Part model, mm, in its own coordinate system. A direction names the side the tool comes from. Give positions to 0.01 mm unless a question says otherwise; leave off trailing zeros. Write each loop counter-clockwise with the first axis right and the second up, starting at its lowest first coordinate (ties: lowest second). Pieces come first, ordered by that corner, then holes. Notation, with made-up numbers: M -33.5,36 L -11.5,36 A12 ccw -11.5,49 Z; hole C 13,-10.5 d1. An arc over 180 degrees is marked long. Use CSV: the item, a comma, the result in double quotes. Start each with the question number.
1. Band-saw the part on A-A, the plane z = -47.5. List the corners of the cut face in (x, y), then the cut area to 3 significant figures.
2. Mould opens along Z. For faces 1 (the face through (-76.986, 2.465, 77.297)), 2 (the face through (-1, 2, 95)), 3 (the face through (-88.866, 2.535, 73.953)), 4 (the face through (-1, 2, -95)) say: pulls with the +Z half, pulls with the -Z half, needs draft (parallel to the pull), parting line crosses it, or undercut.
3. Band-saw the part on B-B, the plane x = -54.5. List the corners of the cut face in (y, z).
4. Band-saw the part on C-C, the plane y = 4.05. Count the separate pieces of the cut face and the enclosed holes in it, then the cut area to 3 significant figures.
5. 3-axis set-ups, long thin cutter, end or side, ignore diameter. For faces 5 (the face through (-90, 2, -90)), 6 (the face through (83, 3, 1)): which of +Z, -Z, +X, -X, +Y, -Y reach the whole face in a straight line?
6. Band-saw the part on D-D, the plane x = -89. List the corners of the cut face in (y, z), then the cut area to 4 significant figures.
7. Drill centre lines: line 1 along Z through (x, y) = (-31.5, 3.4); line 2 along X through (y, z) = (1.65, 64); line 3 along X through (y, z) = (3.5, -77). Where is each one in solid material? Low to high. Write a range as from..to.
from build123d import *

# Parameters (mm, degrees)
SKETCH1_W           = 190
SKETCH1_H           = 190
BOSS_EXTRUDE1_DEPTH = 5
SKETCH2_W           = 166
SKETCH2_H           = 166
CUT_EXTRUDE1_DEPTH  = 135.443296597
FILLET1_R           = 20
SKETCH3_R           = 3.05
CUT_EXTRUDE2_DEPTH  = 135.443296597
SKETCH4_R           = 3.05
CUT_EXTRUDE3_DEPTH  = 10
CHAMFER1_SIZE       = 10


with BuildPart() as part:
    # Sketch1 → Boss-Extrude1 (new body)
    with BuildSketch(Plane(origin=(0, 0, 0), x_dir=(1, 0, 0), z_dir=(0, 1, 0))):
        Rectangle(SKETCH1_W, SKETCH1_H)
    extrude(amount=BOSS_EXTRUDE1_DEPTH)

    # Sketch2 → Cut-Extrude1 (cut, through all)
    with BuildSketch(Plane(origin=(0, 5, 0), x_dir=(1, 0, 0), z_dir=(0, 1, 0))):
        Rectangle(SKETCH2_W, SKETCH2_H)
    extrude(amount=-CUT_EXTRUDE1_DEPTH, mode=Mode.SUBTRACT)

    # Fillet1
    fillet1_edges = [part.edges().sort_by_distance(p)[0] for p in [
        (83, 2.5, -83),
        (83, 2.5, 83),
        (-83, 2.5, 83),
        (-83, 2.5, -83),
    ]]
    fillet(fillet1_edges, radius=FILLET1_R)

    # Sketch3 → Cut-Extrude2 (cut, through all)
    with BuildSketch(Plane(origin=(0, 5, 0), x_dir=(1, 0, 0), z_dir=(0, 1, 0))):
        with Locations(Location((-77, 89, 0), (0, 0, 270))):
            Circle(SKETCH3_R)
        with Locations(Location((-89, 68, 0), (0, 0, 270))):
            Circle(SKETCH3_R)
        with Locations(Location((89, 77, 0), (0, 0, 270))):
            Circle(SKETCH3_R)
        with Locations(Location((68, 89, 0), (0, 0, 270))):
            Circle(SKETCH3_R)
        with Locations(Location((77, -89, 0), (0, 0, 270))):
            Circle(SKETCH3_R)
        with Locations(Location((89, -68, 0), (0, 0, 270))):
            Circle(SKETCH3_R)
        with Locations(Location((-89, -77, 0), (0, 0, 270))):
            Circle(SKETCH3_R)
        with Locations(Location((-68, -89, 0), (0, 0, 270))):
            Circle(SKETCH3_R)
    extrude(amount=-CUT_EXTRUDE2_DEPTH, mode=Mode.SUBTRACT)

    # Sketch4 → Cut-Extrude3 (cut)
    with BuildSketch(Plane(origin=(0, 5, 0), x_dir=(1, 0, 0), z_dir=(0, 1, 0))):
        with Locations(Location((-89, 3, 0), (0, 0, 270))):
            Circle(SKETCH4_R)
        with Locations(Location((89, 12, 0), (0, 0, 270))):
            Circle(SKETCH4_R)
    extrude(amount=-CUT_EXTRUDE3_DEPTH, mode=Mode.SUBTRACT)

    # Chamfer1
    chamfer1_edges = [part.edges().sort_by_distance(p)[0] for p in [
        (-95, 2.5, -95),
        (-95, 2.5, 95),
        (95, 2.5, 95),
        (95, 2.5, -95),
    ]]
    chamfer(chamfer1_edges, length=CHAMFER1_SIZE)


solid = part.part
Output:
1,outline,"M -95,0 L -83,0 L -83,5 L -95,5 Z; M 83,0 L 95,0 L 95,5 L 83,5 Z"
1,area,"120 mm²"
2,face 1,"undercut"
2,face 2,"pulls with the +Z half"
2,face 3,"undercut"
2,face 4,"pulls with the -Z half"
3,outline,"M 0,-95 L 5,-95 L 5,-83 L 0,-83 Z; M 0,83 L 5,83 L 5,95 L 0,95 Z"
4,separate pieces,"1"
4,enclosed holes,"11"
4,area,"8,400 mm²"
5,face 5,"-Z, -X, +Y, -Y"
5,face 6,"+Y, -Y"
6,outline,"M 0,-91 L 5,-91 L 5,-71.05 L 0,-71.05 Z; M 0,-64.95 L 5,-64.95 L 5,-6.05 L 0,-6.05 Z; M 0,0.05 L 5,0.05 L 5,73.95 L 0,73.95 Z; M 0,80.05 L 5,80.05 L 5,91 L 0,91 Z"
6,area,"818.5 mm²"
7,line 1,"z = -95..-83, 83..95"
7,line 2,"x = -95..-82.97, 82.97..95"
7,line 3,"x = -95..-77.28, 77.28..85.95, 92.05..95"
